Geometry check sheet. Reference: the model listing, model coordinates, mm. Face numbers are marked on the shaded views. A direction names the side the tool comes from. Give positions to 0.01 mm unless a question says otherwise; leave off trailing zeros. Loops run counter-clockwise (first coordinate to the right, second up) from the corner with the lowest first, then second, coordinate; pieces in that order, holes last. Notation, with made-up numbers: (65, 35) -> (80, 35) arc R25 cw to (80, 49) -> close; hole circle Ø8 at (24.5, 62). An arc over 180 degrees is marked (long way). Write item = value, one per line.
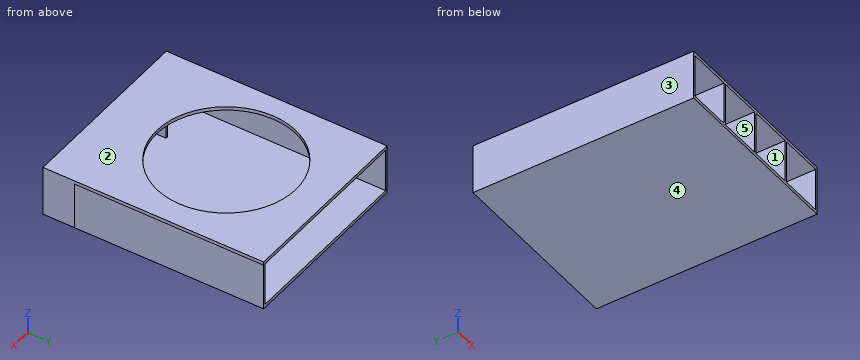
```python
from build123d import *

# Parameters (mm, degrees)
F0_W     = 147.32
F0_H     = 40.513
F0_W_2   = 1.524
F0_H_2   = 34.925
F1_DEPTH = 25.4
F2_W     = 1.5239988621
F2_H     = 34.925
F2_W_2   = 1.5240011379
F3_DEPTH = 152.4
F4_R     = 55.88
F5_DEPTH = 25.4


with BuildPart() as f1:
    # F0 (on Front) → F1 (new body)
    with BuildSketch(Plane.XZ):
        with Locations((22.8904561008, 15.2461919377)):
            Rectangle(F0_W, F0_H)
        Polygon((-49.2455427613, 32.7086919377), (-14.3205427613, 32.7086919377), (-12.7965427613, 32.7086919377), (22.1284572387, 32.7086919377), (23.6524572387, 32.7086919377), (58.5774572387, 32.7086919377), (60.1014572387, 32.7086919377), (95.0264572387, 32.7086919377), (95.0264572387, -2.2163080623), (60.1014572387, -2.2163080623), (58.5774572387, -2.2163080623), (23.6524572387, -2.2163080623), (22.1284572387, -2.2163080623), (-12.7965427613, -2.2163080623), (-14.3205427613, -2.2163080623), (-49.2455427613, -2.2163080623), align=None, mode=Mode.SUBTRACT)
        with Locations((-13.5585427613, 15.2461919377)):
            Rectangle(F0_W_2, F0_H_2)
        with Locations((22.8904572387, 15.2461919377)):
            Rectangle(F0_W_2, F0_H_2)
        with Locations((59.3394572387, 15.2461919377)):
            Rectangle(F0_W_2, F0_H_2)
    extrude(amount=-F1_DEPTH)

    # F2 (on face) → F3 (join)
    with BuildSketch(Plane(origin=(0, 25.4, 0), x_dir=(-1, 0, 0), z_dir=(0, 1, 0))):
        with Locations((-95.7884566697, 15.2461919377)):
            Rectangle(F2_W, F2_H)
        Polygon((-60.1014572387, -2.2163080623), (-95.0264572387, -2.2163080623), (-96.5504561008, -2.2163080623), (-96.5504561008, -5.0103080623), (50.7695438992, -5.0103080623), (50.7695438992, -2.2163080623), (49.2455427613, -2.2163080623), (14.3205427613, -2.2163080623), (12.7965427613, -2.2163080623), (-22.1284572387, -2.2163080623), (-23.6524572387, -2.2163080623), (-58.5774572387, -2.2163080623), align=None)
        Polygon((-96.5504561008, 32.7086919377), (-95.0264572387, 32.7086919377), (-60.1014572387, 32.7086919377), (-58.5774572387, 32.7086919377), (-23.6524572387, 32.7086919377), (-22.1284572387, 32.7086919377), (12.7965427613, 32.7086919377), (14.3205427613, 32.7086919377), (49.2455427613, 32.7086919377), (50.7695438992, 32.7086919377), (50.7695438992, 35.5026919377), (-96.5504561008, 35.5026919377), align=None)
        with Locations((50.0075433303, 15.2461919377)):
            Rectangle(F2_W_2, F2_H)
    extrude(amount=F3_DEPTH)

    # F4 (on face) → F5 (cut)
    with BuildSketch(Plane.XY.offset(35.5026919377)):
        with Locations((21.5660557151, 97.1244573593)):
            Circle(F4_R)
    extrude(amount=-F5_DEPTH, mode=Mode.SUBTRACT)


solid = f1.part
```
Item 1: Tool access check on the marked faces 4 and 5. Record the directions out of +Z, -Z, +X, -X, +Y, -Y that give a thin tool (end or side, any length) a straight path to the whole face; none if there is none.
Answer:
face_4 = -Z, +X, -X, +Y, -Y
face_5 = +Y, -Y
Item 2: Section check D-D, the plane y = 134.5. Record the cut outline in (x, z).
Answer:
outline = (-50.77, -5.01) -> (96.55, -5.01) -> (96.55, 35.5) -> (63.11, 35.5) -> (63.11, 32.71) -> (95.03, 32.71) -> (95.03, -2.22) -> (-49.25, -2.22) -> (-49.25, 32.71) -> (-19.97, 32.71) -> (-19.97, 35.5) -> (-50.77, 35.5) -> close
Item 3: Section check C-C, the plane x = 75.5. Record the cut outline in (y, z).
Answer:
outline = (0, -5.01) -> (177.8, -5.01) -> (177.8, -2.22) -> (0, -2.22) -> close; (0, 32.71) -> (82.51, 32.71) -> (82.51, 35.5) -> (0, 35.5) -> close; (111.74, 32.71) -> (177.8, 32.71) -> (177.8, 35.5) -> (111.74, 35.5) -> close
Item 4: Section check B-B, the plane y = 167.5. Record the cut outline in (x, z), plus the area to 3 significant figures.
Answer:
outline = (-50.77, -5.01) -> (96.55, -5.01) -> (96.55, 35.5) -> (-50.77, 35.5) -> close; hole (-49.25, -2.22) -> (95.03, -2.22) -> (95.03, 32.71) -> (-49.25, 32.71) -> close
area = 930 mm^2
Item 5: Draft check along Z on the marked faces 1, 2 and 3. Enter one of: +Z half, -Z half, draft (parallel to the pull), parting line (faces both ways), or undercut.
Answer:
face_1 = undercut
face_2 = +Z half
face_3 = draft
Item 6: Section check A-A, the plane z = 29. Record the cut outline in (x, y).
Answer:
outline = (-50.77, 0) -> (-49.25, 0) -> (-49.25, 177.8) -> (-50.77, 177.8) -> close; (-14.32, 0) -> (-12.8, 0) -> (-12.8, 25.4) -> (-14.32, 25.4) -> close; (22.13, 0) -> (23.65, 0) -> (23.65, 25.4) -> (22.13, 25.4) -> close; (58.58, 0) -> (60.1, 0) -> (60.1, 25.4) -> (58.58, 25.4) -> close; (95.03, 0) -> (96.55, 0) -> (96.55, 177.8) -> (95.03, 177.8) -> close
Item 7: Thickness scan on L1, parallel to X at y = 8.5, z = 27; L2, parallel to X at y = 36.5, z = 18; L3, parallel to Z at x = -14.5, y = 18.5. Record the ranges inside material, lowest first. Write a range as [from, to].
Answer:
L1 = [-50.77, -49.25], [-14.32, -12.8], [22.13, 23.65], [58.58, 60.1], [95.03, 96.55]
L2 = [-50.77, -49.25], [95.03, 96.55]
L3 = [-5.01, -2.22], [32.71, 35.5]
Item 8: Gauge pin test, flat ends, axial feed: pin 1 (2 mm diameter, centred on x = 9, z = -0.5, fed in from -Y) (1 decimal); pin 2 (1.2 mm diameter, centred on x = 22.5, z = 13.5, fed in from +Y). Record the tip position at first contact, or that the pin passes through.
Answer:
pin_1 = through
pin_2 = 25.4
